from build123d import *

# Parameters (mm, degrees)
SKETCH1_R           = 1.4
BOSS_EXTRUDE1_DEPTH = 4
SKETCH2_R           = 1.4
BOSS_EXTRUDE2_DEPTH = 4
SKETCH3_W           = 35.8
SKETCH3_H           = 38.5
BOSS_EXTRUDE3_DEPTH = 6
CUT_EXTRUDE1_DEPTH  = 3.5
SKETCH5_R           = 1.7
CUT_EXTRUDE3_DEPTH  = 67.053160409


with BuildPart() as part:
    # Sketch1 → Boss-Extrude1 (new body)
    with BuildSketch(Plane(origin=(0, 0, 0), x_dir=(1, 0, 0), z_dir=(0, 1, 0))):
        Polygon((-17.9, 45), (-17.9, -5.6), (17.9, -5.6), (17.9, 45), (12.3, 45), (12.3, 0), (-12.3, 0), (-12.3, 45), align=None)
        with Locations(Location((-8.5, -2.8, 0), (0, 0, 270))):
            Circle(SKETCH1_R, mode=Mode.SUBTRACT)
        with Locations(Location((8.5, -2.8, 0), (0, 0, 90))):
            Circle(SKETCH1_R, mode=Mode.SUBTRACT)
        with Locations(Location((15.1, 37.5, 0), (0, 0, 270))):
            Circle(SKETCH1_R, mode=Mode.SUBTRACT)
        with Locations(Location((15.1, 20.5, 0), (0, 0, 270))):
            Circle(SKETCH1_R, mode=Mode.SUBTRACT)
        with Locations(Location((15.1, 3.5, 0), (0, 0, 270))):
            Circle(SKETCH1_R, mode=Mode.SUBTRACT)
        with Locations(Location((-15.1, 3.5, 0), (0, 0, 90))):
            Circle(SKETCH1_R, mode=Mode.SUBTRACT)
        with Locations(Location((-15.1, 20.5, 0), (0, 0, 90))):
            Circle(SKETCH1_R, mode=Mode.SUBTRACT)
        with Locations(Location((-15.1, 37.5, 0), (0, 0, 90))):
            Circle(SKETCH1_R, mode=Mode.SUBTRACT)
    extrude(amount=BOSS_EXTRUDE1_DEPTH)



with BuildPart() as body_2:
    # Sketch2 → Boss-Extrude2 (new body)
    with BuildSketch(Plane(origin=(0, 34.5, 0), x_dir=(1, 0, 0), z_dir=(0, 1, 0))):
        Polygon((-17.9, -5.6), (17.9, -5.6), (17.9, 45), (12.3, 45), (12.3, 0), (-12.3, 0), (-12.3, 45), (-17.9, 45), align=None)
        with Locations(Location((8.5, -2.8, 0), (0, 0, 90))):
            Circle(SKETCH2_R, mode=Mode.SUBTRACT)
        with Locations(Location((-8.5, -2.8, 0), (0, 0, 270))):
            Circle(SKETCH2_R, mode=Mode.SUBTRACT)
        with Locations(Location((-15.1, 3.5, 0), (0, 0, 90))):
            Circle(SKETCH2_R, mode=Mode.SUBTRACT)
        with Locations(Location((-15.1, 20.5, 0), (0, 0, 90))):
            Circle(SKETCH2_R, mode=Mode.SUBTRACT)
        with Locations(Location((15.1, 3.5, 0), (0, 0, 270))):
            Circle(SKETCH2_R, mode=Mode.SUBTRACT)
        with Locations(Location((15.1, 20.5, 0), (0, 0, 270))):
            Circle(SKETCH2_R, mode=Mode.SUBTRACT)
        with Locations(Location((15.1, 37.5, 0), (0, 0, 270))):
            Circle(SKETCH2_R, mode=Mode.SUBTRACT)
        with Locations(Location((-15.1, 37.5, 0), (0, 0, 90))):
            Circle(SKETCH2_R, mode=Mode.SUBTRACT)
    extrude(amount=BOSS_EXTRUDE2_DEPTH)


with BuildPart() as part_1:
    add(part.part)

    add(body_2.part)  # Boss-Extrude3 merges body 2
    # Sketch3 → Boss-Extrude3 (add)
    with BuildSketch(Plane.XY.offset(5.6)):
        with Locations((0, 19.25)):
            Rectangle(SKETCH3_W, SKETCH3_H)
    extrude(amount=BOSS_EXTRUDE3_DEPTH)

    # Sketch4 → Cut-Extrude1 (cut)
    with BuildSketch(Plane(origin=(0, 0, 5.6), x_dir=(-1, 0, 0), z_dir=(0, 0, -1))):
        Polygon((8.325684219, 26.35), (6.651368439, 29.25), (8.325684219, 32.15), (11.674315781, 32.15), (13.348631561, 29.25), (11.674315781, 26.35), align=None)
        Polygon((-8.325684219, 26.35), (-6.651368439, 29.25), (-8.325684219, 32.15), (-11.674315781, 32.15), (-13.348631561, 29.25), (-11.674315781, 26.35), align=None)
        Polygon((6.651368439, 9.25), (8.325684219, 6.35), (11.674315781, 6.35), (13.348631561, 9.25), (11.674315781, 12.15), (8.325684219, 12.15), align=None)
        Polygon((-6.651368439, 9.25), (-8.325684219, 6.35), (-11.674315781, 6.35), (-13.348631561, 9.25), (-11.674315781, 12.15), (-8.325684219, 12.15), align=None)
    extrude(amount=-CUT_EXTRUDE1_DEPTH, mode=Mode.SUBTRACT)

    # Sketch5 → Cut-Extrude3 (cut, through all)
    with BuildSketch(Plane(origin=(0, 0, 5.6), x_dir=(-1, 0, 0), z_dir=(0, 0, -1))):
        with Locations((-10, 29.25)):
            Circle(SKETCH5_R)
        with Locations((-10, 9.25)):
            Circle(SKETCH5_R)
        with Locations((10, 9.25)):
            Circle(SKETCH5_R)
        with Locations((10, 29.25)):
            Circle(SKETCH5_R)
    extrude(amount=-CUT_EXTRUDE3_DEPTH, mode=Mode.SUBTRACT)


solid = part_1.part
Verification items for the finished model (mm, model axes). A direction names the side the tool comes from. Give positions to 0.01 mm unless a question says otherwise; leave off trailing zeros. Loops run counter-clockwise (first coordinate to the right, second up) from the corner with the lowest first, then second, coordinate; pieces in that order, holes last. Notation, with made-up numbers: (19.5, 68.25) - (61.5, 68.25) arc R22 cw to (61.5, 74.25) - close; hole circle Ø2 at (-14.75, -27). An arc over 180 degrees is marked (long way). Write each question's results on one line, items separated by ' | '.
1) Sectioned sample at B-B on z = -10.5. Record the boundary of the cut face in (x, y), plus the area to 3 significant figures.
Solution:
outline: (-17.9, 0) - (-12.3, 0) - (-12.3, 4) - (-17.9, 4) - close; (-17.9, 34.5) - (-12.3, 34.5) - (-12.3, 38.5) - (-17.9, 38.5) - close; (12.3, 0) - (17.9, 0) - (17.9, 4) - (12.3, 4) - close; (12.3, 34.5) - (17.9, 34.5) - (17.9, 38.5) - (12.3, 38.5) - close | area: 89.6 mm2
2) Mould release check, pull along X, two halves, no side actions. Record for faces 1 (the flat face through (15, 2, -45)), 2 (the cylindrical face through (14.56, 1.97, -36.21)): pulls with the +X half, pulls with the -X half, needs draft (parallel to the pull), parting line crosses it, or undercut.
Solution:
face 1: needs draft | face 2: undercut
3) Sectioned sample at C-C on z = 2.8. Record the boundary of the cut face in (x, y), plus the area to 3 significant figures.
Solution:
outline: (-17.9, 0) - (-9.9, 0) - (-9.9, 4) - (-17.9, 4) - close; (-17.9, 34.5) - (-9.9, 34.5) - (-9.9, 38.5) - (-17.9, 38.5) - close; (-7.1, 0) - (7.1, 0) - (7.1, 4) - (-7.1, 4) - close; (-7.1, 34.5) - (7.1, 34.5) - (7.1, 38.5) - (-7.1, 38.5) - close; (9.9, 0) - (17.9, 0) - (17.9, 4) - (9.9, 4) - close; (9.9, 34.5) - (17.9, 34.5) - (17.9, 38.5) - (9.9, 38.5) - close | area: 242 mm2
4) Tool access check on faces 3 (the flat face through (-12.3, 2, -22)), 4 (the flat face through (10, 26.35, 7)), 5 (the flat face through (-13, 34.5, -12)), 6 (the flat face through (0, 0, 4)). Record the directions out of +Z, -Z, +X, -X, +Y, -Y that give a thin tool (end or side, any length) a straight path to the whole face; none if there is none.
Solution:
face 3: -Z, +Y, -Y | face 4: -Z | face 5: -Z, +X, -X | face 6: +Z, -Z, +X, -X, -Y
5) Sectioned sample at A-A on x = -15.1. Count the separate pieces of the cut face and the enclosed holes in it, plus the area to 3 significant figures.
Solution:
separate pieces: 7 | enclosed holes: 0 | area: 569 mm2
6) Depth check by flat-ended pin: P1, Ø12, axis at y = 12, z = -2, coming from the -X side; P2, Ø4.5, axis at x = -2.5, y = 35.5, coming from the -Z side; P3, Ø1, axis at x = -12, y = 15.5, coming from the -Z side. Enter the tip coordinate at first touch or a pass-through.
Solution:
P1: through | P2: z = 0 | P3: z = 5.6
7) Material ranges on L1, parallel to Z at x = -15.1, y = 36.6; L2, parallel to Y at x = -10, z = 10.9; L3, parallel to X at y = 2.2, z = 2.8, recorded low to high. Write a range as from..to.
Solution:
L1: -45..-38.9, -36.1..-21.9, -19.1..-4.9, -2.1..11.6 | L2: 0..7.55, 10.95..27.55, 30.95..38.5 | L3: -17.9..-9.9, -7.1..7.1, 9.9..17.9
